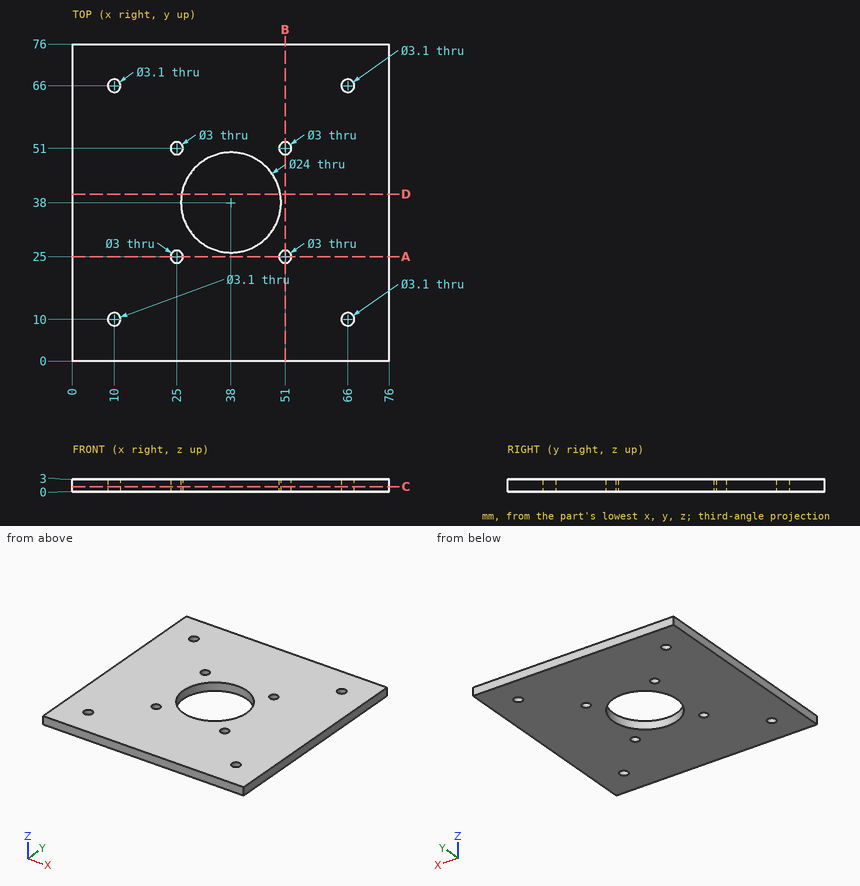
Could you check a few things on this drawing? It's one solid part, dimensions in mm from its lowest x, y, z. Give positions to 0.01 mm unless a question says otherwise; leave off trailing zeros. Order: outer loops, then holes, each group sorted by start corner. A loop starts at its lowest first (then second) coordinate and runs counter-clockwise, first axis right, second up. Notation, with made-up numbers: (46.25, 5.25) - (71.25, 5.25) arc R15 ccw to (71.25, 28.25) - close; hole circle Ø1 at (-21, 62.5). An arc over 180 degrees is marked (long way). One line per item, written item: value. Start each with the question number.
1. Imagine slicing it at D-D on y = 40. List the corners of the cut face in (x, z) for me.
2. If I drill on probe 1 along Y at (x, z) = (66, 2.6); probe 2 along Y at (x, z) = (50.5, 0.2); probe 3 along X at (y, z) = (52, 1.55), over which ranges is the centre line in solid material (lowest first)?
3. Imagine slicing it at C-C on z = 1.15. Give the number of separate pieces and of enclosed holes in the cut face, plus the area to 3 significant figures.
4. Imagine slicing it at A-A on y = 25. List the corners of the cut face in (x, z) for me, plus the area to 3 significant figures.
5. For P1, Ø4, axis at x = 10, y = 10, coming from the -Z side, with a flat end and sliding along its axis, tell me the tip position at first contact or that it passes through.
Values:
1. outline: (0, 0) - (26.17, 0) - (26.17, 3) - (0, 3) - close; (49.83, 0) - (76, 0) - (76, 3) - (49.83, 3) - close
2. probe 1: 0 to 8.45, 11.55 to 64.45, 67.55 to 76
2. probe 2: 0 to 23.59, 26.41 to 49.59, 52.41 to 76
2. probe 3: 0 to 23.88, 26.12 to 49.88, 52.12 to 76
3. separate pieces: 1
3. enclosed holes: 9
3. area: 5,270 mm²
4. outline: (0, 0) - (23.5, 0) - (23.5, 3) - (0, 3) - close; (26.5, 0) - (49.5, 0) - (49.5, 3) - (26.5, 3) - close; (52.5, 0) - (76, 0) - (76, 3) - (52.5, 3) - close
4. area: 210 mm²
5. P1: z = 0
